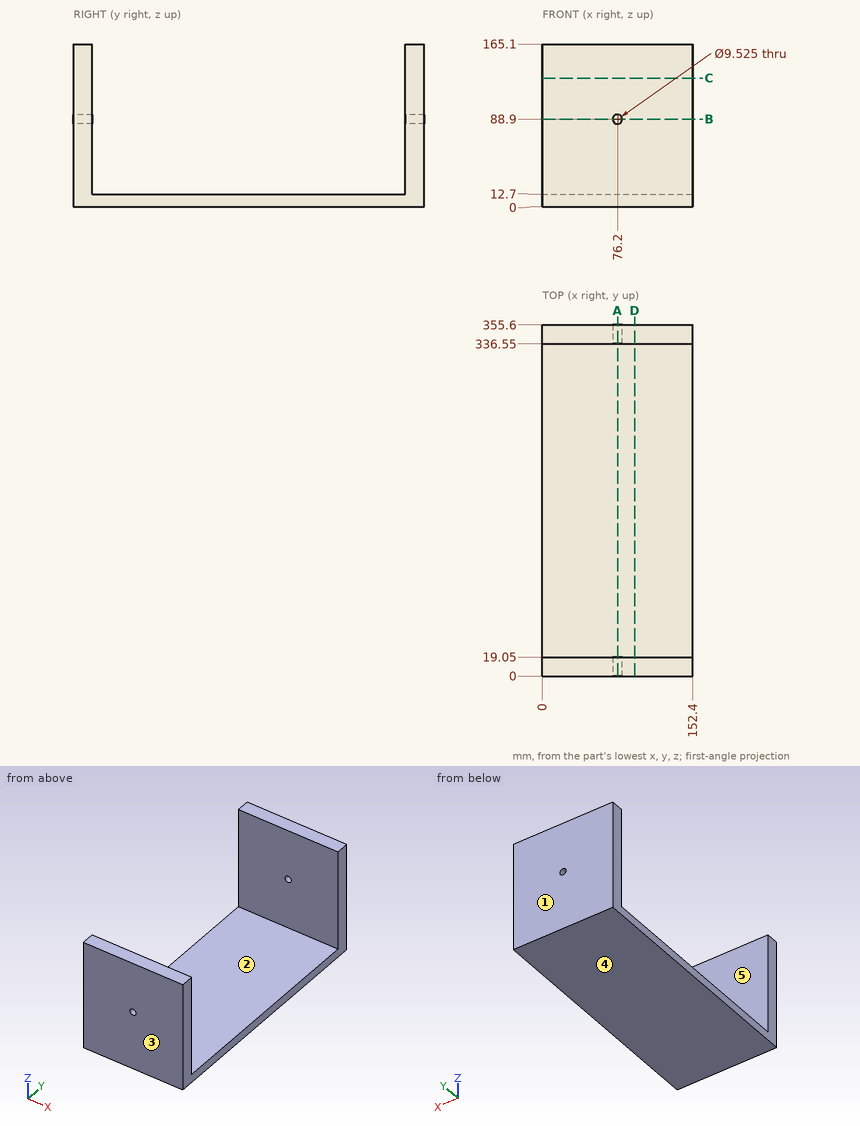
Input: dimensioned drawing with shaded views. Units: mm. Origin: part minimum x, y, z. A direction names the side the tool comes from. Round coordinates to 2 decimals unless told otherwise and drop trailing zeros. Write each loop counter-clockwise with the first axis right and the second up, starting at its lowest first coordinate (ties: lowest second). Pieces come first, ordered by that corner, then holes. Notation, with made-up numbers: (-11.5, -18.5) - (27.5, -18.5) arc R17 cw to (27.5, 4.5) - close; hole circle Ø3 at (76.25, 83.25). An arc over 180 degrees is marked (long way). Write item = value, one per line.
(1) Contact query for a flat-ended pin moving along its axis: pin 1 Ø8.5 at (x, z) = (76.2, 88.9) entering from -Y. Output: stop coordinate, or through.
Geometry check:
pin_1 = through
(2) Section query A-A on x = 76.2. Output: boundary loops of the cut face in (y, z).
Geometry check:
outline = (0, 0) - (355.6, 0) - (355.6, 84.14) - (336.55, 84.14) - (336.55, 12.7) - (19.05, 12.7) - (19.05, 84.14) - (0, 84.14) - close; (0, 93.66) - (19.05, 93.66) - (19.05, 165.1) - (0, 165.1) - close; (336.55, 93.66) - (355.6, 93.66) - (355.6, 165.1) - (336.55, 165.1) - close
(3) Section query B-B on z = 88.9. Output: boundary loops of the cut face in (x, y), then the cut area to 3 significant figures.
Geometry check:
outline = (0, 0) - (71.44, 0) - (71.44, 19.05) - (0, 19.05) - close; (0, 336.55) - (71.44, 336.55) - (71.44, 355.6) - (0, 355.6) - close; (80.96, 0) - (152.4, 0) - (152.4, 19.05) - (80.96, 19.05) - close; (80.96, 336.55) - (152.4, 336.55) - (152.4, 355.6) - (80.96, 355.6) - close
area = 5,440 mm^2
(4) Section query C-C on z = 130.5. Output: boundary loops of the cut face in (x, y).
Geometry check:
outline = (0, 0) - (152.4, 0) - (152.4, 19.05) - (0, 19.05) - close; (0, 336.55) - (152.4, 336.55) - (152.4, 355.6) - (0, 355.6) - close
(5) Access query for the marked faces 1 and 2. Directions: +Z, -Z, +X, -X, +Y, -Y. A direction counts if a zero-diameter tool reaches every point of the face in a straight line with its end or side. Return the directions, or none.
Geometry check:
face_1 = +Z, -Z, +X, -X, +Y
face_2 = +Z, +X, -X
(6) Material intervals for probe 1 along Y at (x, z) = (99.5, 99.5); probe 2 along Z at (x, y) = (76.2, 342.25), sorted ascending.
Geometry check:
probe_1 = 0 to 19.05, 336.55 to 355.6
probe_2 = 0 to 84.14, 93.66 to 165.1
(7) Pull-direction query (Y, two-part tool) for the marked faces 3, 4 and 5; classes: +Y half, -Y half, draft (parallel to the pull), parting line (faces both ways), or undercut.
Geometry check:
face_3 = -Y half
face_4 = draft
face_5 = undercut
(8) Section query D-D on x = 93.5. Output: boundary loops of the cut face in (y, z), then the cut area to 3 significant figures.
Geometry check:
outline = (0, 0) - (355.6, 0) - (355.6, 165.1) - (336.55, 165.1) - (336.55, 12.7) - (19.05, 12.7) - (19.05, 165.1) - (0, 165.1) - close
area = 10,300 mm^2
